```python
from build123d import *

# Parameters (mm, degrees)
F0_W     = 88.9
F0_H     = 44.45
F1_DEPTH = 50.8
F3_D     = 6.7564
F4_R     = 6.35


with BuildPart() as f1:
    # F0 (on Top) → F1 (new body)
    with BuildSketch(Plane.XY):
        Rectangle(F0_W, F0_H)
    extrude(amount=F1_DEPTH)

    # F3 (through all)
    with Locations(Plane(origin=(0, 22.225, 0), x_dir=(-1, 0, 0), z_dir=(0, 1, 0))):
        with Locations((-19.05, 25.4), (19.05, 25.4)):
            Hole(F3_D / 2)

    # F4
    f4_edges = [f1.edges().sort_by_distance(p)[0] for p in [
        (0, 22.225, 50.8),
        (-44.45, 22.225, 25.4),
        (0, 22.225, 0),
        (44.45, 22.225, 25.4),
    ]]
    fillet(f4_edges, radius=F4_R)


solid = f1.part
```
Work out the finished part from the listing and answer in its coordinate system (mm). Give positions to 0.01 mm unless a question says otherwise; leave off trailing zeros. Loops run counter-clockwise (first coordinate to the right, second up) from the corner with the lowest first, then second, coordinate; pieces in that order, holes last. Notation, with made-up numbers: M -5.5,-16 L 11.5,-16 A29 ccw 11.5,13 Z; hole C 64.25,-39 d4. An arc over 180 degrees is marked long. One line per item, written item: value. Start each with the question number.
1. Find the intervals of material crossed by probe 1 along X at (y, z) = (-5, 25); probe 2 along Z at (x, y) = (-19.05, -6.5); probe 3 along X at (y, z) = (-0.5, 23.5), in increasing order.
2. Find section A-A (x = -19.05). Give the vertices of the cut face in (y, z) (3 decimals).
3. Find section C-C (y = 2). Give the vertices of the cut face in (x, z).
4. Determine the mould class of faces 1 (the face through (-19.78, -0.31, 22.1)), 2 (the face through (-44.45, -3, 25)), 3 (the face through (20.6, -0.3, 22.4)), 4 (the face through (0.622, 20.414, 48.89)) for opening direction Z: released by +Z, released by -Z, zero draft, split by the parting line, or undercut.
5. Find section B-B (z = 25.4). Give the vertices of the cut face in (x, y) (3 decimals).
Reported:
1. probe 1: x = -44.45 to -22.4, -15.7 to 15.7, 22.4 to 44.45
1. probe 2: z = 0 to 22.02, 28.78 to 50.8
1. probe 3: x = -44.45 to -21.84, -16.26 to 16.26, 21.84 to 44.45
2. outline: M -22.225,0 L 15.875,0 A6.35 ccw 22.225,6.35 L 22.225,22.022 L -22.225,22.022 Z; M -22.225,28.778 L 22.225,28.778 L 22.225,44.45 A6.35 ccw 15.875,50.8 L -22.225,50.8 Z
3. outline: M -44.45,0 L 44.45,0 L 44.45,50.8 L -44.45,50.8 Z; hole C -19.05,25.4 d6.76; hole C 19.05,25.4 d6.76
4. face 1: undercut
4. face 2: zero draft
4. face 3: undercut
4. face 4: released by +Z
5. outline: M -44.45,-22.225 L -22.428,-22.225 L -22.428,22.225 L -38.1,22.225 A6.35 ccw -44.45,15.875 Z; M -15.672,-22.225 L 15.672,-22.225 L 15.672,22.225 L -15.672,22.225 Z; M 22.428,-22.225 L 44.45,-22.225 L 44.45,15.875 A6.35 ccw 38.1,22.225 L 22.428,22.225 Z
